Answer from the drawing. Dimensions are ordinates in mm from the lowest x, y and z of the part. Coordinates: 2 decimals unless noted, no trailing zeros. Write each loop counter-clockwise with the first axis right and the second up, starting at its lowest first coordinate (ties: lowest second). Pieces come first, ordered by that corner, then holes. Notation, with made-up numbers: (88, 1) - (146, 1) arc R19 cw to (146, 7) - close; hole circle Ø5 at (-37.5, -11.75). An arc over 180 degrees is marked (long way). Use one line per item in the form item = value. Start each with the question number.
Item 1: Given pin 1 (2.5 mm diameter, centred on x = 79, y = 42, fed in from -Z), flat-ended and moving along its own axis, determine where the tip first touches the part or whether it passes through.
Item 2: A cutting plane is placed at D-D (y = 73.5). Write down the section's boundary in (x, z).
Item 3: Consider probe 1 along Y at (x, z) = (11, 1.5) (1 decimal); probe 2 along Y at (x, z) = (29.5, 2.55) (1 decimal); probe 3 along Y at (x, z) = (41, 1.3). Determine where each line is inside the solid, lowest interval first.
Item 4: A cutting plane is placed at C-C (z = 0.85). Give the number of separate pieces and of enclosed holes in the cut face, then the cut area to 3 significant figures.
Item 5: A cutting plane is placed at A-A (y = 42). Write down the section's boundary in (x, z).
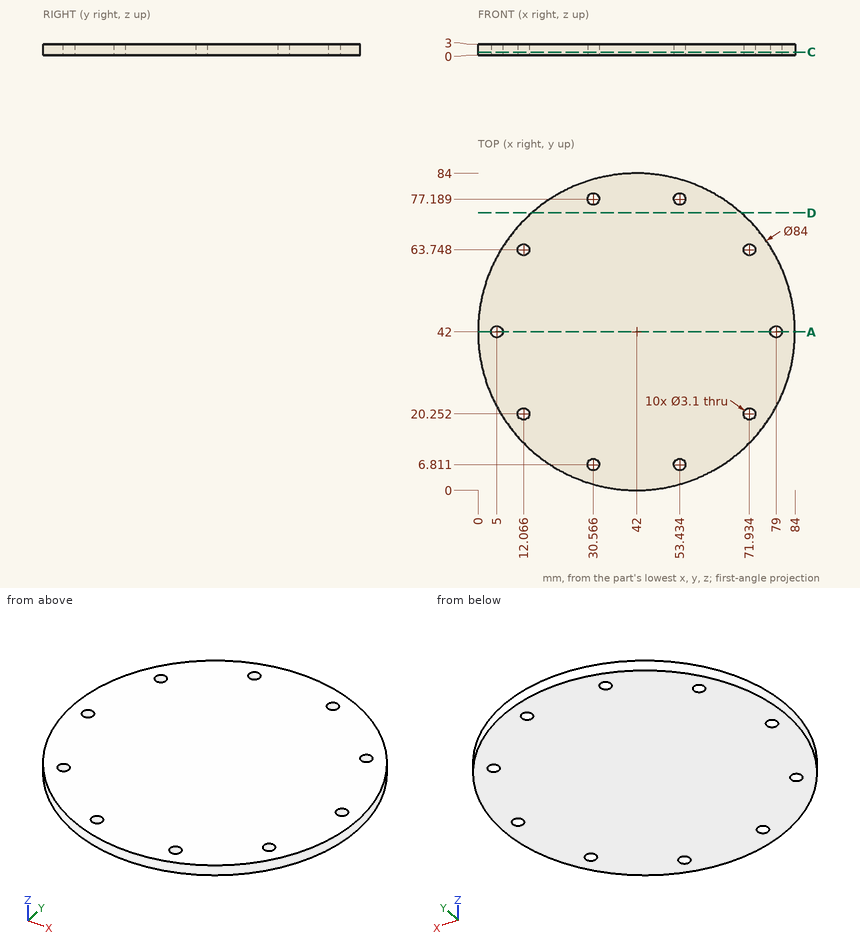
Answer:
q1.pin_1 = through
q2.outline = (14.22, 0) - (69.78, 0) - (69.78, 3) - (14.22, 3) - close
q3.probe_1 = 13.7 to 19.1, 21.4 to 62.6, 64.9 to 70.3
q3.probe_2 = 1.9 to 5.7, 7.9 to 76.1, 78.3 to 82.1
q3.probe_3 = 0.01 to 83.99
q4.separate_pieces = 1
q4.enclosed_holes = 10
q4.area = 5,470 mm²
q5.outline = (0, 0) - (3.45, 0) - (3.45, 3) - (0, 3) - close; (6.55, 0) - (77.45, 0) - (77.45, 3) - (6.55, 3) - close; (80.55, 0) - (84, 0) - (84, 3) - (80.55, 3) - close
